For this review, take the finished solid that the model builds, in its own axes (mm). Coordinates: 2 decimals unless noted, no trailing zeros. Loops run counter-clockwise (first coordinate to the right, second up) from the corner with the lowest first, then second, coordinate; pieces in that order, holes last. Notation, with made-up numbers: M 47.5,32.5 L 61.5,32.5 A20 cw 61.5,44.5 Z; hole C 10.5,8 d6. An arc over 180 degrees is marked long. Answer as a JSON object with one key per item and string values. Group by question number.
Item 1: Add section C-C (y = 1.35). Count the separate pieces of the cut face and the enclosed holes in it, then the cut area to 3 significant figures.
Item 2: Wall thickness on L1, parallel to Z at x = -17, y = 2.15; L2, parallel to X at y = 3.35, z = 0; L3, parallel to X at y = 1.3, z = -43: over which ranges is each line inside the solid? List them lowest first. Write a range as from..to.
Item 3: Add section A-A (x = 0). State the section outline as (y, z) points, then the cut area to 3 significant figures.
Item 4: Insertion check: pin 1 (3 mm diameter, centred on x = 13, z = 17, fed in from +Y). The pin has a flat end and moves straight along its axis. Give the tip position at first contact, or say it passes through.
Item 5: Mouldability with a two-part tool opening along X and no side actions: class faces 1 (the face through (11, 3, 18.5)), 2 (the face through (53, 3, -39)), 3 (the face through (-26.14, 3.04, 26.1)), 4 (the face through (12, 3, -103)) as +X half, -X half, draft (parallel to the pull), parting line (faces both ways), or undercut.
Item 6: Add section D-D (x = -17). State the section outline as (y, z) points.
Item 7: Add section B-B (z = -43). State the section outline as (x, y) points, then the cut area to 3 significant figures.
from build123d import *

# Parameters (mm, degrees)
SKETCH1_W           = 80
SKETCH1_H           = 130
SKETCH1_R           = 2
SKETCH1_R_2         = 2.5
BOSS_EXTRUDE1_DEPTH = 6
FILLET1_R           = 3


with BuildPart() as part:
    # Sketch1 → Boss-Extrude1 (new body)
    with BuildSketch(Plane(origin=(0, 0, 0), x_dir=(1, 0, 0), z_dir=(0, 1, 0))):
        with Locations((13, 38)):
            Rectangle(SKETCH1_W, SKETCH1_H)
        with Locations((0, 26)):
            Circle(SKETCH1_R, mode=Mode.SUBTRACT)
        with Locations((26, 26)):
            Circle(SKETCH1_R, mode=Mode.SUBTRACT)
        with Locations((26, 0)):
            Circle(SKETCH1_R, mode=Mode.SUBTRACT)
        Circle(SKETCH1_R, mode=Mode.SUBTRACT)
        with Locations((-17, 43)):
            Circle(SKETCH1_R_2, mode=Mode.SUBTRACT)
        with Locations((43, 43)):
            Circle(SKETCH1_R_2, mode=Mode.SUBTRACT)
        with Locations((43, -17)):
            Circle(SKETCH1_R_2, mode=Mode.SUBTRACT)
        with Locations((-17, -17)):
            Circle(SKETCH1_R_2, mode=Mode.SUBTRACT)
        with Locations((13, 43)):
            Circle(SKETCH1_R_2, mode=Mode.SUBTRACT)
        with Locations((13, -17)):
            Circle(SKETCH1_R_2, mode=Mode.SUBTRACT)
    extrude(amount=BOSS_EXTRUDE1_DEPTH)

    # Fillet1
    fillet1_edges = [part.edges().sort_by_distance(p)[0] for p in [
        (53, 3, 27),
        (-27, 3, 27),
    ]]
    fillet(fillet1_edges, radius=FILLET1_R)


solid = part.part
From the geometry:
{
 "1": {"separate pieces": "1", "enclosed holes": "10", "area": "10,200 mm²"},
 "2": {"L1": "z = -103..-45.5, -40.5..14.5, 19.5..27", "L2": "x = -27..-2, 2..24, 28..53", "L3": "x = -27..-19.5, -14.5..10.5, 15.5..40.5, 45.5..53"},
 "3": {"outline": "M 0,-103 L 6,-103 L 6,-28 L 0,-28 Z; M 0,-24 L 6,-24 L 6,-2 L 0,-2 Z; M 0,2 L 6,2 L 6,27 L 0,27 Z", "area": "732 mm²"},
 "4": {"pin 1": "passes through"},
 "5": {"face 1": "undercut", "face 2": "+X half", "face 3": "-X half", "face 4": "draft"},
 "6": {"outline": "M 0,-103 L 6,-103 L 6,-45.5 L 0,-45.5 Z; M 0,-40.5 L 6,-40.5 L 6,14.5 L 0,14.5 Z; M 0,19.5 L 6,19.5 L 6,27 L 0,27 Z"},
 "7": {"outline": "M -27,0 L -19.5,0 L -19.5,6 L -27,6 Z; M -14.5,0 L 10.5,0 L 10.5,6 L -14.5,6 Z; M 15.5,0 L 40.5,0 L 40.5,6 L 15.5,6 Z; M 45.5,0 L 53,0 L 53,6 L 45.5,6 Z", "area": "390 mm²"}
}
